```python
from build123d import *

# Parameters (mm, degrees)
CUT_EXTRUDE1_DEPTH      = 58.445626622
CUT_EXTRUDE1_DEPTH_BACK = 10
SKETCH3_R               = 10
FILLET4_R               = 5
FILLET5_R               = 2


with BuildPart() as part:
    # Loft1: read off the stored shape, not the designer's step
    # Loft1: loft between two sections, ruled curve by curve
    loft1_from = [
        Edge.make_bspline([(-10.493972108, 50, -10.718047835), (10.942123561, 50, -31.705992052), (31.930067778, 50, -10.269896382), (10.493972108, 50, 10.718047835), (-10.942123561, 50, 31.705992052), (-31.930067778, 50, 10.269896382), (-10.493972108, 50, -10.718047835)], [0, 0, 0, 0, 0.5, 0.5, 0.5, 1, 1, 1, 1], 3, [1, 0.333333333, 0.333333333, 1, 0.333333333, 0.333333333, 1]),
    ]
    loft1_to = [
        Edge.make_bspline([(-17.436793853, 0, -9.795826669), (2.154859485, 0, -44.669414375), (37.028447191, 0, -25.077761037), (17.436793853, 0, 9.795826669), (-2.154859485, 0, 44.669414375), (-37.028447191, 0, 25.077761037), (-17.436793853, 0, -9.795826669)], [0, 0, 0, 0, 0.5, 0.5, 0.5, 1, 1, 1, 1], 3, [1, 0.333333333, 0.333333333, 1, 0.333333333, 0.333333333, 1]),
    ]
    loft1 = Solid(Shell([*[Face.make_surface_from_curves(loft1_from[k], loft1_to[k]) for k in range(1)], Face(Wire(loft1_from)), Face(Wire(loft1_to))]))
    add(loft1)

    # Sketch3 → Cut-Extrude1 (cut, two sides: drawn at the far end of the back side and taken through both)
    with BuildSketch(Plane(origin=(0, 50, 0), x_dir=(1, 0, 0), z_dir=(0, 1, 0)).offset(-CUT_EXTRUDE1_DEPTH_BACK)):
        with Locations(Location((0, 0, 0), (0, 0, 270))):
            Circle(SKETCH3_R)
    extrude(amount=CUT_EXTRUDE1_DEPTH + CUT_EXTRUDE1_DEPTH_BACK, mode=Mode.SUBTRACT)

    # Fillet4
    fillet4_edges = [part.edges().sort_by_distance(p)[0] for p in [
        (17.436793853, 0, 9.795826669),
    ]]
    fillet(fillet4_edges, radius=FILLET4_R)

    # Fillet5
    fillet5_edges = [part.edges().sort_by_distance(p)[0] for p in [
        (10.493972108, 50, 10.718047835),
        (0, 50, -10),
    ]]
    fillet(fillet5_edges, radius=FILLET5_R)


solid = part.part
```
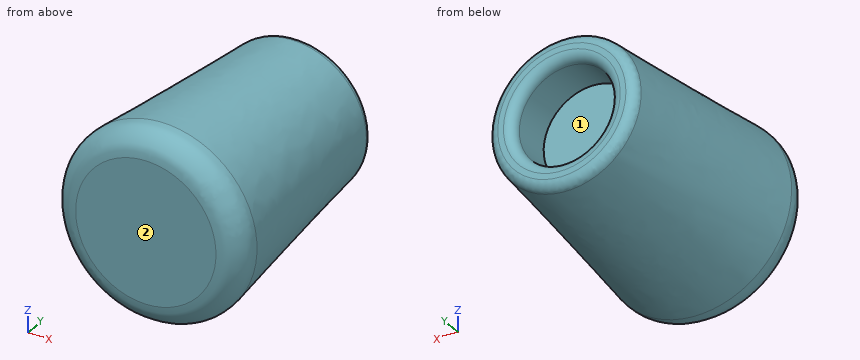
Build history of the part. All positions in model axes, mm. Face numbers are marked on the shaded views. Round coordinates to 2 decimals unless told otherwise and drop trailing zeros. Use a Markdown table: item, result.
1) Flat gauge pins, fed straight in: pin 1 Ø6 at (y, z) = (23.5, -5.5) entering from -X; pin 2 Ø12 at (y, z) = (9.5, -3) entering from -X; pin 3 Ø1.5 at (x, y) = (8, 24.5) entering from +Z; pin 4 Ø1.5 at (x, y) = (7.5, 11) entering from -Z. Where does each tip first touch, or does it go through?
Recorded:
| item | result |
|---|---|
| pin 1 | stops at x = -17.39 |
| pin 2 | stops at x = -19.41 |
| pin 3 | stops at z = 15.8 |
| pin 4 | stops at z = -17.55 |
2) Wall check: L1, parallel to X at y = 46.25, z = 0; L2, parallel to X at y = 43.5, z = 0; L3, parallel to Z at x = 0, y = 44.5. Give the ranges that are in metal, low to high.
Recorded:
| item | result |
|---|---|
| L1 | x = -15.32 to -10, 10 to 15.32 |
| L2 | x = -15.56 to -10, 10 to 15.56 |
| L3 | z = -15.47 to -10, 10 to 15.47 |
3) Pull direction X, two halves, no side cores. Call the marked faces 1 and 2: pulls with the +X half, pulls with the -X half, needs draft (parallel to the pull), parting line crosses it, or undercut.
Recorded:
| item | result |
|---|---|
| face 1 | undercut |
| face 2 | needs draft |
